Build history of the part. All positions in model axes, mm. A direction names the side the tool comes from. Give positions to 0.01 mm unless a question says otherwise; leave off trailing zeros. Loops run counter-clockwise (first coordinate to the right, second up) from the corner with the lowest first, then second, coordinate; pieces in that order, holes last. Notation, with made-up numbers: (15, 62) - (23, 62) arc R18 ccw to (23, 81) - close; hole circle Ø5 at (9.25, 70). An arc over 180 degrees is marked (long way). Return JSON: item names as keys, results as strings. Group by question number.
1) Slice it at D-D (y = -17.5). List the corners of the cut face in (x, z), and give its area (3 significant figures).
2) Mould opens along X. For faces 3 (the face through (-1, -6, 0)), 4 (the face through (1.232, -9.538, 42.954)), 5 (the face through (-9, 2, 0)), 6 (the face through (0, -9.8, 43.1)) say: released by +X, released by -X, zero draft, split by the parting line, or undercut.
3) Drop flat-ended pins along their axis: pin 1 (8 mm diameter, centred on x = -5.5, y = -1, fed in from +Z); pin 2 (5 mm diameter, centred on x = 0.5, z = -20.5, fed in from +Y); pin 3 (6 mm diameter, centred on x = -1, z = 24, fed in from +Y). Give the stop position or say it passes through.
4) Drill centre lines: probe 1 along X at (y, z) = (-19, 40); probe 2 along Z at (x, y) = (-3, 0) (3 decimals); probe 3 along Y at (x, z) = (2.75, -22). Where is each one in solid material? Low to high. Write a range as from..to.
5) 3-axis set-ups, long thin cutter, end or side, ignore diameter. For faces 1 (the face through (1.219, 29.041, 29.646)), 2 (the face through (3.5, 0, -3)): which of +Z, -Z, +X, -X, +Y, -Y reach the whole face in a straight line?
6) Slice it at C-C (z = -24). List the corners of the cut face in (x, y).
7) Slice it at A-A (z = 0). List the corners of the cut face in (x, y) (3 decimals), and give its area (3 significant figures).
Autodesk Inventor part; units mm, degrees
ref_plane "YZ Plane" through (0, 0, 0) normal (1, 0, 0) x (0, 1, 0)
ref_plane "XZ Plane" through (0, 0, 0) normal (0, 1, 0) x (-1, 0, 0)
ref_plane "XY Plane" through (0, 0, 0) normal (0, 0, 1) x (1, 0, 0)
sketch "Sketch1" plane through (0, 0, 0) normal (1, 0, 0) x (0, 1, 0)
  circle A0 centre (0, 0) radius 44
  dimension "d0" = 88
extrude "Extrusion1" add sketch "Sketch1" along normal blind 3.5
sketch "Sketch2" plane through (3.5, 0, 0) normal (1, 0, 0) x (0, 0, -1)
  circle A0 centre (0, 0) radius 45
  dimension "d3" = 90
extrude "Extrusion2" add sketch "Sketch2" along normal blind 1
sketch "Sketch3" plane through (0, 0, 0) normal (-1, 0, 0) x (0, 0, 1)
  circle A0 centre (0, 0) radius 45
  dimension "d6" = 90
extrude "Extrusion3" add sketch "Sketch3" along normal blind 1
sketch "Sketch4" plane through (4.5, 0, 0) normal (1, 0, 0) x (0, 0, -1)
  circle A0 centre (0, 0) radius 41.5
  dimension "d9" = 83
extrude "Extrusion4" cut sketch "Sketch4" against normal blind 6
sketch "Sketch5" plane through (4.5, 0, 0) normal (1, 0, 0) x (0, 0, -1)
  circle A0 centre (0, 0) radius 3.5
  dimension "d12" = 7
extrude "Extrusion5" add sketch "Sketch5" against normal blind 10
sketch "Sketch6" plane through (4.5, 0, 0) normal (1, 0, 0) x (0, 0, -1)
  circle A0 centre (0, 0) radius 45
extrude "Extrusion6" cut sketch "Sketch6" against normal blind 2
sketch "Sketch7" plane through (2.5, 0, 0) normal (1, 0, 0) x (0, 0, -1)
  circle A0 centre (0, 0) radius 3.5
  circle A1 centre (0, 0) radius 41.5
  circle A2 centre (0, 0) radius 45
extrude "Extrusion7" add sketch "Sketch7" along normal blind 1 contours A2
sketch "Sketch8" plane through (2.5, 0, 0) normal (1, 0, 0) x (0, 0, -1)
  circle A0 centre (0, 0) radius 3.5
extrude "Extrusion8" add sketch "Sketch8" along normal blind 1
sketch "Sketch9" plane through (3.5, 0, 0) normal (1, 0, 0) x (0, 0, -1)
  circle A0 centre (0, 0) radius 1.625
  dimension "d21" = 3.25
extrude "Extrusion9" cut sketch "Sketch9" against normal blind 10
sketch "Sketch10" plane through (3.5, 0, 0) normal (1, 0, 0) x (0, 0, -1)
  line L0 (2, 2.1756) -> (-2, 2.1756)
  line L1 (-2, 2.1756) -> (-2, 42.8244)
  line L2 (-2, 42.8244) -> (2, 42.8244)
  line L3 (2, 42.8244) -> (2, 2.1756)
  line L4 (2, 2.1756) -> (-2, 42.8244) construction
  line L5 (-2, 2.1756) -> (2, 42.8244) construction
  point P0 (0, 0)
  point P1 (0, 22.5)
  dimension "d24" = 4
extrude "Extrusion10" add sketch "Sketch10" against normal blind 4.5
pattern_circular "Circular Pattern1" count 4 over 360 about axis through (4.5, 0, 0) along (-1, 0, 0) of "Extrusion10"
fillet "Fillet1" radius 2 5 edges at (-1, 0, 3.5) (-1, -3.5, 0) (-1, 3.5, 0) (-1, -1.0481, -3.3394) (-1, 1.0481, -3.3394)
sketch "Sketch11" plane through (-5.5, 0, 0) normal (-1, 0, 0) x (0, 0, 1)
  circle A0 centre (0, 0) radius 1.625
  circle A1 centre (0, 0) radius 3.5
extrude "Extrusion11" add sketch "Sketch11" along normal blind 2
sketch "Sketch12" plane through (-7.5, 0, 0) normal (-1, 0, 0) x (0, 0, 1)
  circle A0 centre (0, 0) radius 1.625
  circle A1 centre (0, 0) radius 2
  dimension "d33" = 4
extrude "Extrusion12" add sketch "Sketch12" along normal blind 3.3
properties part number "mtv_pushingWheel_2-25"
Results:
{
 "1": {"outline": "(-1, -41.46) - (0, -41.46) - (0, -40.37) - (2.5, -40.37) - (2.5, -41.46) - (3.5, -41.46) - (3.5, -37.63) - (-1, -37.63) - close; (-1, -2) - (3.5, -2) - (3.5, 2) - (-1, 2) - close; (-1, 37.63) - (3.5, 37.63) - (3.5, 41.46) - (2.5, 41.46) - (2.5, 40.37) - (0, 40.37) - (0, 41.46) - (-1, 41.46) - close", "area": "47.0 mm2"},
 "2": {"face 3": "released by -X", "face 4": "undercut", "face 5": "zero draft", "face 6": "undercut"},
 "3": {"pin 1": "z = 4.11", "pin 2": "y = 41.22", "pin 3": "y = 39.8"},
 "4": {"probe 1": "-1..0, 2.5..3.5", "probe 2": "-3.5..-1.625, 1.625..3.5", "probe 3": "-39.26..-35.19, -2..2, 35.19..39.26"},
 "5": {"face 1": "+X, -X", "face 2": "+Z, -Z, +X, +Y, -Y"},
 "6": {"outline": "(-1, -38.07) - (0, -38.07) - (0, -36.88) - (2.5, -36.88) - (2.5, -38.07) - (3.5, -38.07) - (3.5, -33.86) - (-1, -33.86) - close; (-1, -2) - (3.5, -2) - (3.5, 2) - (-1, 2) - close; (-1, 33.86) - (3.5, 33.86) - (3.5, 38.07) - (2.5, 38.07) - (2.5, 36.88) - (0, 36.88) - (0, 38.07) - (-1, 38.07) - close"},
 "7": {"outline": "(-10.8, -2) - (-7.5, -2) - (-7.5, -3.5) - (-3, -3.5) arc R2 cw to (-1, -5.5) - (-1, -45) - (0, -45) - (0, -44) - (2.5, -44) - (2.5, -45) - (3.5, -45) - (3.5, -1.625) - (-10.8, -1.625) - close; (-10.8, 1.625) - (3.5, 1.625) - (3.5, 45) - (2.5, 45) - (2.5, 44) - (0, 44) - (0, 45) - (-1, 45) - (-1, 5.5) arc R2 cw to (-3, 3.5) - (-7.5, 3.5) - (-7.5, 2) - (-10.8, 2) - close", "area": "414 mm2"}
}
